Model file for the job. Use its own axes, mm. Round coordinates to 2 decimals unless told otherwise and drop trailing zeros. Order: outer loops, then holes, each group sorted by start corner. A loop starts at its lowest first (then second) coordinate and runs counter-clockwise, first axis right, second up. Notation, with made-up numbers: (39.5, 0.25) - (89.5, 0.25) arc R7 cw to (89.5, 13.25) - close; hole circle Ø10 at (10, -7.75). An arc over 180 degrees is marked (long way). Write item = value, one per line.
```python
from build123d import *

# Parameters (mm, degrees)
F1_DEPTH = 76.2
F3_D     = 3.429


with BuildPart() as f1:
    # F0 (on Top) → F1 (new body)
    with BuildSketch(Plane.XY):
        Polygon((-7.306218, 0.126358), (-5.985126, -4.192261), (-2.37792, -6.909579), (2.137572, -6.987673), (5.836583, -4.396713), (7.306218, -0.126358), (5.985126, 4.192261), (2.37792, 6.909579), (-2.137572, 6.987673), (-5.836583, 4.396713), align=None)
    extrude(amount=F1_DEPTH)

    # F3 (through all)
    with Locations(Plane(origin=(0, 0, 0), x_dir=(1, 0, 0), z_dir=(0, 0, -1))):
        with Locations((0, 0)):
            Hole(F3_D / 2)


solid = f1.part
```
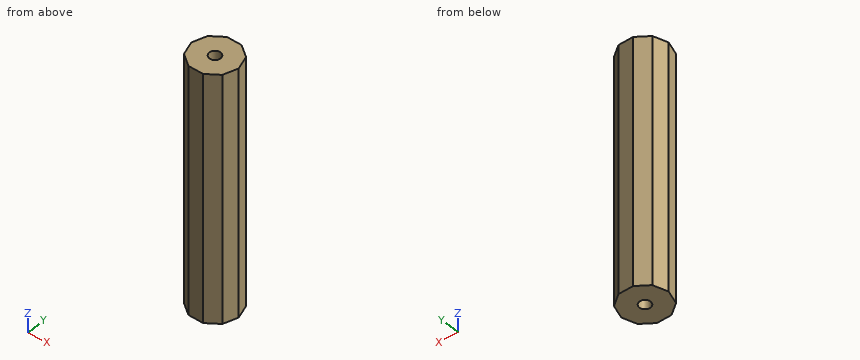
1) Wall check: line 1 along Y through (x, z) = (-1.75, 47); line 2 along Y through (x, z) = (0.5, 58.5); line 3 along Y through (x, z) = (0.25, 14). Give the ranges that are in metal, low to high.
Conclusion:
line_1 = -6.92 to 6.98
line_2 = -6.96 to -1.64, 1.64 to 6.94
line_3 = -6.96 to -1.7, 1.7 to 6.95
2) Cut at D-D (y = 2.5). Write the cut outline in (x, z), and give its area (3 significant figures).
Conclusion:
outline = (-6.49, 0) - (6.5, 0) - (6.5, 76.2) - (-6.49, 76.2) - close
area = 990 mm^2
3) Flat gauge pins, fed straight in: pin 1 Ø5 at (y, z) = (-5.5, 61.5) entering from -X; pin 2 Ø1.5 at (x, z) = (-3, 42) entering from +Y; pin 3 Ø1 at (x, z) = (-4.5, 15.5) entering from +Y. Where does each tip first touch, or does it go through?
Conclusion:
pin_1 = -6.35
pin_2 = 6.91
pin_3 = 5.68
4) Cut at A-A (z = 63.5). Write the cut outline in (x, y).
Conclusion:
outline = (-7.31, 0.13) - (-5.99, -4.19) - (-2.38, -6.91) - (2.14, -6.99) - (5.84, -4.4) - (7.31, -0.13) - (5.99, 4.19) - (2.38, 6.91) - (-2.14, 6.99) - (-5.84, 4.4) - close; hole circle Ø3.43 at (0, 0)
5) Cut at C-C (y = -2.75). Write the cut outline in (x, z), and give its area (3 significant figures).
Conclusion:
outline = (-6.43, 0) - (6.4, 0) - (6.4, 76.2) - (-6.43, 76.2) - close
area = 978 mm^2
6) Cut at B-B (x = 0). Write the cut outline in (y, z), and give its area (3 significant figures).
Conclusion:
outline = (-6.95, 0) - (-1.71, 0) - (-1.71, 76.2) - (-6.95, 76.2) - close; (1.71, 0) - (6.95, 0) - (6.95, 76.2) - (1.71, 76.2) - close
area = 798 mm^2
